Solid Edge part; units mm, degrees
sketch "Sketch1" plane through (0, 0, 0) normal (0, 0, 1) x (1, 0, 0)
  line L0 (-80, -20.75) -> (80, -20.75)
  line L1 (80, -20.75) -> (80, 20.75)
  line L2 (80, 20.75) -> (-80, 20.75)
  line L3 (-80, 20.75) -> (-80, -20.75)
  dimension "D1" = 80
  dimension "D2" = 80
extrude "Protrusion1" add sketch "Sketch1" along normal blind 3
fillet "Round_1" radius 1.5 4 edges at (-80, -20.75, 1.5) (-80, 20.75, 1.5) (80, -20.75, 1.5) (80, 20.75, 1.5)
hole "Hole_1" at (-15.15, 7.45, 3) direction (0, 0, -1) diameter 12 end through all
hole "Hole1" at (1.25, 7.45, 3) direction (0, 0, -1) diameter 12 end through all
hole "Hole2" at (17.8, -6.55, 3) direction (0, 0, -1) diameter 12 end through all
hole "Hole3" at (34.35, 7.45, 3) direction (0, 0, -1) diameter 12 end through all
hole "Hole4" at (50.8, 7.45, 3) direction (0, 0, -1) diameter 12 end through all
hole "Hole5" at (67.15, -6.55, 3) direction (0, 0, -1) diameter 12 end through all
hole "Hole_7" at (75, -15.75, 3) direction (0, 0, -1) diameter 3.2 end up to next countersink diameter 7 countersink angle 90
hole "Hole6" at (75, 13.75, 3) direction (0, 0, -1) diameter 3.2 end up to next countersink diameter 7 countersink angle 90
hole "Hole7" at (-25, -15.75, 3) direction (0, 0, -1) diameter 3.2 end up to next countersink diameter 7 countersink angle 90
hole "Hole8" at (-25, 13.75, 3) direction (0, 0, -1) diameter 3.2 end up to next countersink diameter 7 countersink angle 90
hole "Hole9" at (38, -15.75, 3) direction (0, 0, -1) diameter 3.2 end up to next countersink diameter 7 countersink angle 90
hole "Hole10" at (12, 13.75, 3) direction (0, 0, -1) diameter 3.2 end up to next countersink diameter 7 countersink angle 90
properties material "Stainless Steel, 304"
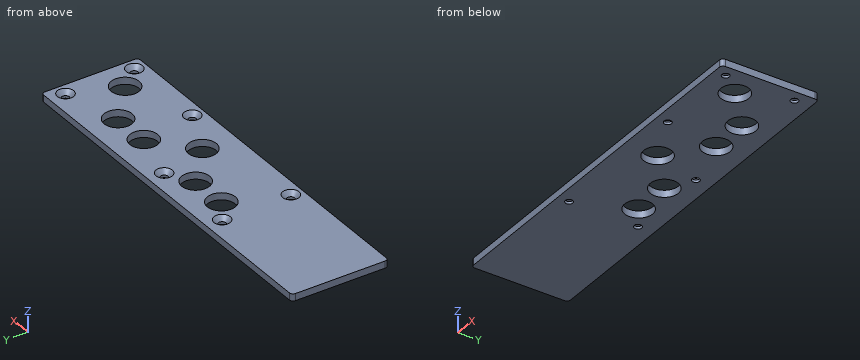
Design review of the part built by this model. Coordinates are the model's own, in mm. Round coordinates to 2 decimals unless told otherwise and drop trailing zeros. Write each loop counter-clockwise with the first axis right and the second up, starting at its lowest first coordinate (ties: lowest second). Pieces come first, ordered by that corner, then holes. Notation, with made-up numbers: (35.5, -7) -> (58.5, -7) arc R25 ccw to (58.5, 7) -> close; hole circle Ø4 at (30, 52). An arc over 180 degrees is marked (long way). Answer in a Markdown table with one row per item.
Q1. To check wall thickness, follow L1, parallel to X at y = -15.75, z = 0.7; L2, parallel to X at y = 13.75, z = 0.35; L3, parallel to X at y = 7.45, z = 1.15. State the ranges of each line that lie inside material, in increasing order. Write a range as [from, to].
The answers:
| item | result |
|---|---|
| L1 | [-80, -26.6], [-23.4, 36.4], [39.6, 73.4], [76.6, 80] |
| L2 | [-80, -26.6], [-23.4, 10.4], [13.6, 73.4], [76.6, 80] |
| L3 | [-80, -21.15], [-9.15, -4.75], [7.25, 28.35], [40.35, 44.8], [56.8, 80] |
Q2. Take a section at B-B, the plane y = -6.55. State the section outline as (x, z) points, then the cut area to 3 significant figures.
The answers:
| item | result |
|---|---|
| outline | (-80, 0) -> (11.8, 0) -> (11.8, 3) -> (-80, 3) -> close; (23.8, 0) -> (61.15, 0) -> (61.15, 3) -> (23.8, 3) -> close; (73.15, 0) -> (80, 0) -> (80, 3) -> (73.15, 3) -> close |
| area | 408 mm² |
Q3. Take a section at D-D, the plane x = -15.15. State the section outline as (y, z) points.
The answers:
| item | result |
|---|---|
| outline | (-20.75, 0) -> (1.45, 0) -> (1.45, 3) -> (-20.75, 3) -> close; (13.45, 0) -> (20.75, 0) -> (20.75, 3) -> (13.45, 3) -> close |
Q4. Clearance check with a flat-ended pin moving along its axis: pin 1 Ø7 at (x, y) = (50.8, 7.45) entering from +Z. State where the tip first meets the part, or that it passes through.
The answers:
| item | result |
|---|---|
| pin 1 | through |
Q5. Take a section at C-C, the plane y = -15.75. State the section outline as (x, z) points.
The answers:
| item | result |
|---|---|
| outline | (-80, 0) -> (-26.6, 0) -> (-26.6, 1.1) -> (-28.5, 3) -> (-80, 3) -> close; (-23.4, 0) -> (36.4, 0) -> (36.4, 1.1) -> (34.5, 3) -> (-21.5, 3) -> (-23.4, 1.1) -> close; (39.6, 0) -> (73.4, 0) -> (73.4, 1.1) -> (71.5, 3) -> (41.5, 3) -> (39.6, 1.1) -> close; (76.6, 0) -> (80, 0) -> (80, 3) -> (78.5, 3) -> (76.6, 1.1) -> close |
Q6. Take a section at A-A, the plane x = 75. State the section outline as (y, z) points, then the cut area to 3 significant figures.
The answers:
| item | result |
|---|---|
| outline | (-20.75, 0) -> (-17.35, 0) -> (-17.35, 1.1) -> (-19.25, 3) -> (-20.75, 3) -> close; (-14.15, 0) -> (12.15, 0) -> (12.15, 1.1) -> (10.25, 3) -> (-12.25, 3) -> (-14.15, 1.1) -> close; (15.35, 0) -> (20.75, 0) -> (20.75, 3) -> (17.25, 3) -> (15.35, 1.1) -> close |
| area | 98.1 mm² |
